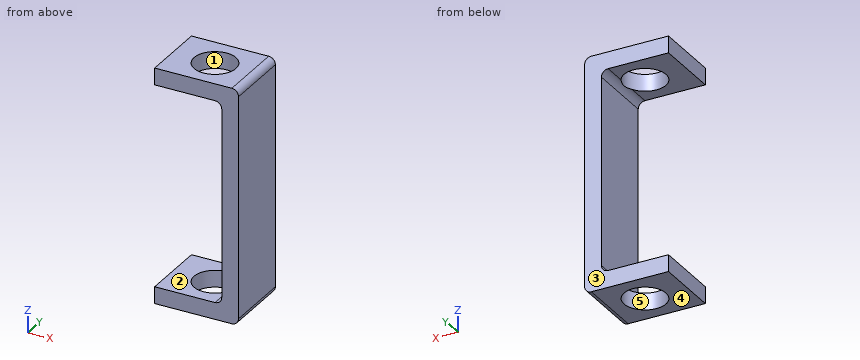
from build123d import *

# Parameters (mm, degrees)
F1_DEPTH = 12.7
F2_R     = 2.54
F3_R     = 7.9375
F4_DEPTH = 127


with BuildPart() as f1:
    # F0 (on Front) → F1 (new body, symmetric)
    with BuildSketch(Plane.XZ):
        Polygon((15.875, 44.45), (-15.875, 44.45), (-15.875, 38.1), (9.525, 38.1), (9.525, -38.1), (-15.875, -38.1), (-15.875, -44.45), (15.875, -44.45), align=None)
    extrude(amount=F1_DEPTH, both=True)

    # F2
    f2_edges = [f1.edges().sort_by_distance(p)[0] for p in [
        (15.875, 0, 44.45),
        (15.875, 0, -44.45),
        (9.525, 0, 38.1),
        (9.525, 0, -38.1),
    ]]
    fillet(f2_edges, radius=F2_R)

    # F3 (on face) → F4 (cut, symmetric)
    with BuildSketch(Plane.XY.offset(44.45)):
        Circle(F3_R)
    extrude(amount=F4_DEPTH, both=True, mode=Mode.SUBTRACT)


solid = f1.part
The listing builds one solid part. Answer for the finished solid, in the listing's coordinates (mm). Face numbers are marked on the shaded views. A direction names the side the tool comes from. Round coordinates to 2 decimals unless told otherwise and drop trailing zeros. Write each loop counter-clockwise with the first axis right and the second up, starting at its lowest first coordinate (ties: lowest second). Pieces come first, ordered by that corner, then holes. Notation, with made-up numbers: (-37.5, 72) - (10.5, 72) arc R27 ccw to (10.5, 106) - close; hole circle Ø6 at (55, -10.75). An arc over 180 degrees is marked (long way). Use one line per item in the form item = value. Start each with the question number.
Item 1: Find the intervals of material crossed by line 1 (Z direction, x = -13, y = -10.25); line 2 (Y direction, x = 0, z = -41); line 3 (X direction, y = 0, z = -42) (1 decimal), in increasing order. Write a range as [from, to].
Item 2: A cutting plane is placed at D-D (z = -33). Write down the section's boundary in (x, y) (3 decimals).
Item 3: A cutting plane is placed at C-C (y = -11). Write down the section's boundary in (x, z) (3 decimals), plus the area to 3 significant figures.
Item 4: Determine the mould class of the marked faces 3, 4 and 5 for opening direction Y: +Y half, -Y half, draft (parallel to the pull), parting line (faces both ways), or undercut.
Item 5: A tool of negligible diameter and unlimited length cuts with its end or side. For the marked faces 1 and 2, from which of +Z, -Z, +X, -X, +Y, -Y can it reach the whole face along a straight path? Write none if from no direction.
Item 6: A flat-ended cylindrical pin translates along its axis: pin 1 Ø2 at (x, y) = (0, -6.5) entering from +Z. Find the tip coordinate at first contact, or state that the pin passes through.
Item 7: A cutting plane is placed at B-B (x = 0). Write down the section's boundary in (y, z).
Item 8: A cutting plane is placed at A-A (y = 0). Give the number of separate pieces and of enclosed holes in the cut face, plus the area to 3 significant figures.
The answers:
q1.line_1 = [-44.45, -38.1], [38.1, 44.45]
q1.line_2 = [-12.7, -7.94], [7.94, 12.7]
q1.line_3 = [-15.9, -7.9], [7.9, 15.9]
q2.outline = (9.525, -12.7) - (15.875, -12.7) - (15.875, 12.7) - (9.525, 12.7) - close
q3.outline = (-15.875, -44.45) - (13.335, -44.45) arc R2.54 ccw to (15.875, -41.91) - (15.875, 41.91) arc R2.54 ccw to (13.335, 44.45) - (-15.875, 44.45) - (-15.875, 38.1) - (6.985, 38.1) arc R2.54 cw to (9.525, 35.56) - (9.525, -35.56) arc R2.54 cw to (6.985, -38.1) - (-15.875, -38.1) - close
q3.area = 887 mm^2
q4.face_3 = +Y half
q4.face_4 = draft
q4.face_5 = undercut
q5.face_1 = +Z, -Z
q5.face_2 = -X, +Y, -Y
q6.pin_1 = through
q7.outline = (-12.7, -44.45) - (-7.94, -44.45) - (-7.94, -38.1) - (-12.7, -38.1) - close; (-12.7, 38.1) - (-7.94, 38.1) - (-7.94, 44.45) - (-12.7, 44.45) - close; (7.94, -44.45) - (12.7, -44.45) - (12.7, -38.1) - (7.94, -38.1) - close; (7.94, 38.1) - (12.7, 38.1) - (12.7, 44.45) - (7.94, 44.45) - close
q8.separate_pieces = 3
q8.enclosed_holes = 0
q8.area = 685 mm^2
